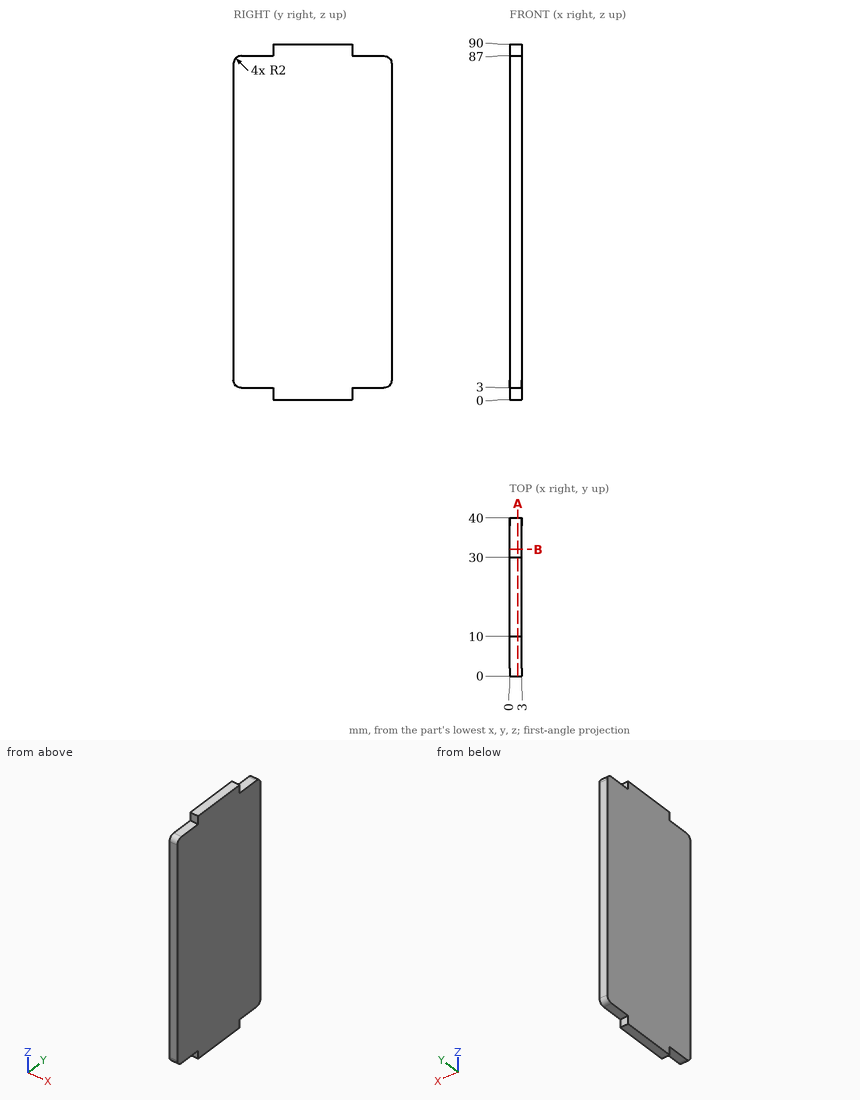
Check sheet for the drawn part. Datum: minimum x, y, z corner. Units: mm. Round coordinates to 2 decimals unless told otherwise and drop trailing zeros. Write each loop counter-clockwise with the first axis right and the second up, starting at its lowest first coordinate (ties: lowest second). Pieces come first, ordered by that corner, then holes. Notation, with made-up numbers: (-12, -11.75) -> (19, -11.75) arc R18 ccw to (19, 4.25) -> close; hole circle Ø4 at (84.25, 22.5). An arc over 180 degrees is marked (long way). Put each result on its own line as item: value.
(1) Go/stop test with flat-tipped pins: pin 1 Ø1.5 at (x, y) = (1, 32.5) entering from -Z; pin 2 Ø0.9 at (x, z) = (2, 88) entering from -Y. Record where each tip stops, or that it passes through.
Values found:
pin 1: stops at z = 3
pin 2: stops at y = 10
(2) Sectioned sample at B-B (y = 32). Enter the section's corners in (x, z).
Values found:
outline: (0, 3) -> (3, 3) -> (3, 87) -> (0, 87) -> close
(3) Material ranges on line 1 (Z direction, x = 2.65, y = 35), recorded low to high.
Values found:
line 1: z = 3 to 87
(4) Sectioned sample at A-A (x = 2.1). Enter the section's corners in (y, z), plus the area to 3 significant figures.
Values found:
outline: (0, 5) arc R2 ccw to (2, 3) -> (10, 3) -> (10, 0) -> (30, 0) -> (30, 3) -> (38, 3) arc R2 ccw to (40, 5) -> (40, 85) arc R2 ccw to (38, 87) -> (30, 87) -> (30, 90) -> (10, 90) -> (10, 87) -> (2, 87) arc R2 ccw to (0, 85) -> close
area: 3,480 mm^2
